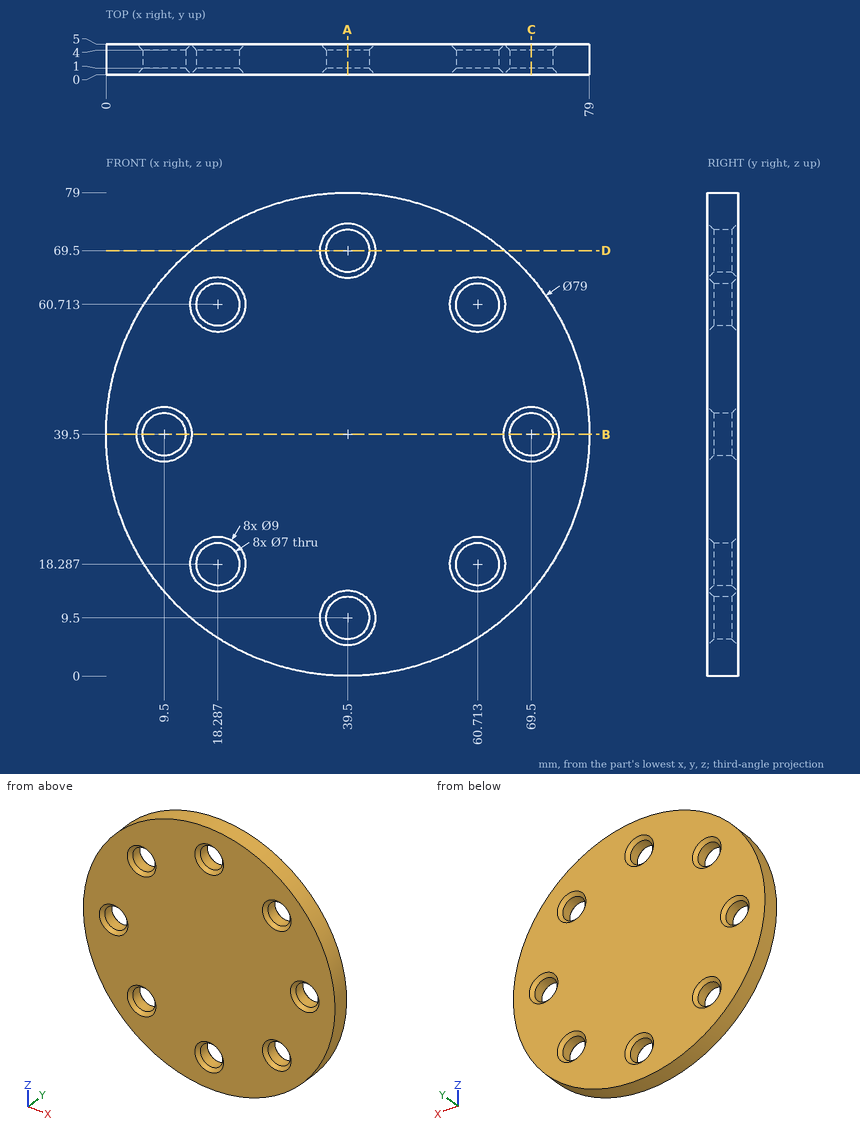
Check sheet for the drawn part. Datum: minimum x, y, z corner. Units: mm. Give positions to 0.01 mm unless a question says otherwise; leave off trailing zeros. Order: outer loops, then holes, each group sorted by start corner. A loop starts at its lowest first (then second) coordinate and runs counter-clockwise, first axis right, second up. Notation, with made-up numbers: (64.5, 56.5) -> (97.5, 56.5) arc R15 cw to (97.5, 68.5) -> close; hole circle Ø5 at (-22, 65.25). An arc over 180 degrees is marked (long way). Use a Markdown table: item, result.
1) Section check D-D, the plane z = 69.5. Record the boundary of the cut face in (x, y) (1 decimal).
Results:
| item | result |
|---|---|
| outline | (13.8, 0) -> (35, 0) -> (36, 1) -> (36, 4) -> (35, 5) -> (13.8, 5) -> close; (43, 1) -> (44, 0) -> (65.2, 0) -> (65.2, 5) -> (44, 5) -> (43, 4) -> close |
2) Material ranges on probe 1 along Z at (x, y) = (15.5, 3.8) (1 decimal); probe 2 along Z at (x, y) = (41, 1); probe 3 along X at (y, z) = (2.3, 17) (1 decimal), recorded low to high.
Results:
| item | result |
|---|---|
| probe 1 | 8.1 to 16.2, 20.4 to 58.6, 62.8 to 70.9 |
| probe 2 | 0.03 to 6.34, 12.66 to 66.34, 72.66 to 78.97 |
| probe 3 | 7 to 15, 21.5 to 57.5, 64 to 72 |
3) Section check C-C, the plane x = 69.5. Record the boundary of the cut face in (y, z) (1 decimal), then the cut area to 3 significant figures.
Results:
| item | result |
|---|---|
| outline | (0, 13.8) -> (5, 13.8) -> (5, 35) -> (4, 36) -> (1, 36) -> (0, 35) -> close; (0, 44) -> (1, 43) -> (4, 43) -> (5, 44) -> (5, 65.2) -> (0, 65.2) -> close |
| area | 220 mm² |
4) Section check A-A, the plane x = 39.5. Record the boundary of the cut face in (y, z), then the cut area to 3 significant figures.
Results:
| item | result |
|---|---|
| outline | (0, 0) -> (5, 0) -> (5, 5) -> (4, 6) -> (1, 6) -> (0, 5) -> close; (0, 14) -> (1, 13) -> (4, 13) -> (5, 14) -> (5, 65) -> (4, 66) -> (1, 66) -> (0, 65) -> close; (0, 74) -> (1, 73) -> (4, 73) -> (5, 74) -> (5, 79) -> (0, 79) -> close |
| area | 321 mm² |
5) Section check B-B, the plane z = 39.5. Record the boundary of the cut face in (x, y).
Results:
| item | result |
|---|---|
| outline | (0, 0) -> (5, 0) -> (6, 1) -> (6, 4) -> (5, 5) -> (0, 5) -> close; (13, 1) -> (14, 0) -> (65, 0) -> (66, 1) -> (66, 4) -> (65, 5) -> (14, 5) -> (13, 4) -> close; (73, 1) -> (74, 0) -> (79, 0) -> (79, 5) -> (74, 5) -> (73, 4) -> close |
6) Depth check by flat-ended pin: pin 1 Ø8 at (x, z) = (69.5, 39.5) entering from +Y; pin 2 Ø1 at (y, z) = (3.5, 70) entering from +X (1 decimal); pin 3 Ø8 at (x, z) = (60.71, 18.29) entering from -Y (1 decimal). Enter the tip coordinate at first touch or a pass-through.
Results:
| item | result |
|---|---|
| pin 1 | y = 4.5 |
| pin 2 | x = 65.2 |
| pin 3 | y = 0.5 |
